The listing builds one solid part. Answer for the finished solid, in the listing's coordinates (mm). Coordinates: 2 decimals unless noted, no trailing zeros. Write each loop counter-clockwise with the first axis right and the second up, starting at its lowest first coordinate (ties: lowest second). Pieces come first, ordered by that corner, then holes. Notation, with made-up numbers: M -4,0.5 L 37,0.5 A16 cw 37,18.5 Z; hole C 0,48 d6. An arc over 180 degrees is marked long. Answer as a JSON object with one key per item and string values. Group by question number.
Autodesk Inventor part; units mm, degrees
ref_plane "YZ Plane" through (0, 0, 0) normal (1, 0, 0) x (0, 1, 0)
ref_plane "XZ Plane" through (0, 0, 0) normal (0, 1, 0) x (-1, 0, 0)
ref_plane "XY Plane" through (0, 0, 0) normal (0, 0, 1) x (1, 0, 0)
sketch "Sketch1" plane through (0, 0, 0) normal (0, 1, 0) x (-1, 0, 0)
  line L0 (0, 0) -> (0, -212.266) construction
  line L1 (-3, 0) -> (-3, -212.266)
  line L2 (3, -212.266) -> (3, 0)
  arc A0 (3, 0) -> (-3, 0) centre (0, 0) ccw
  arc A1 (-3, -212.266) -> (3, -212.266) centre (0, -212.266) ccw
  circle A2 centre (0, 0) radius 1.5
  circle A3 centre (0, -212.266) radius 1.5
  circle A4 centre (0, -72.721) radius 1.5
  arc A5 (3, -25) -> (3, -69.721) centre (79.8115, -47.3605) ccw
  arc A6 (-3, -25) -> (-3, -69.721) centre (73.8115, -47.3605) ccw
  point P0 (0, -106.133)
  dimension "d0" = 6
  dimension "d1" = 212.266
  dimension "d2" = 3
  dimension "d3" = 3
  dimension "d10" = 3
  dimension "d11" = 72.721
  dimension "d12" = 80
  dimension "d13" = 80
  dimension "d14" = 3
  dimension "d15" = 25
extrude "Extrusion1" add sketch "Sketch1" along normal blind 10 contours A0 L2 A5 A1 L1 | L1 A6
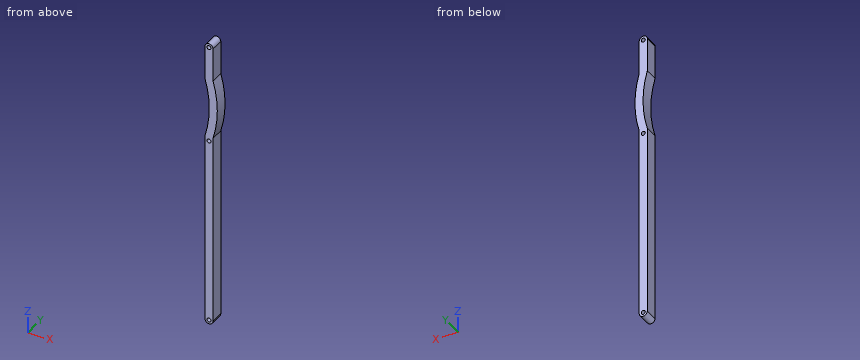
Item 1: Flat-ended cylindrical pins translate along their axes: pin 1 Ø3 at (y, z) = (9, -85) entering from +X; pin 2 Ø2 at (x, y) = (-1.5, 6) entering from +Z. Find the tip coordinate at first contact, or state that the pin passes through.
Item 2: Consider L1, parallel to Z at x = 1.25, y = 9.5; L2, parallel to X at y = 2.5, z = -177; L3, parallel to X at y = 7.25, z = -47.5. Determine where each line is inside the solid, lowest interval first. Write a range as from..to.
Item 3: A cutting plane is placed at B-B, the plane z = -198.5. Write down the section's boundary in (x, y), and give its area (3 significant figures).
Item 4: A cutting plane is placed at A-A, the plane y = 4.5. Write down the section's boundary in (x, z), and give its area (3 significant figures).
Answer:
{
 "1": {"pin 1": "x = 3", "pin 2": "z = 2.96"},
 "2": {"L1": "-214.99..-213.1, -211.44..-73.55, -71.89..-0.83, 0.83..2.73", "L2": "-3..3", "L3": "0.19..6.19"},
 "3": {"outline": "M -3,0 L 3,0 L 3,10 L -3,10 Z", "area": "60.0 mm2"},
 "4": {"outline": "M -3,-212.27 A3 ccw 3,-212.27 L 3,-69.72 A80 ccw 3,-25 L 3,0 A3 ccw -3,0 L -3,-25 A80 cw -3,-69.72 Z; hole C 0,-212.27 d3; hole C 0,-72.72 d3; hole C 0,0 d3", "area": "1,280 mm2"}
}
